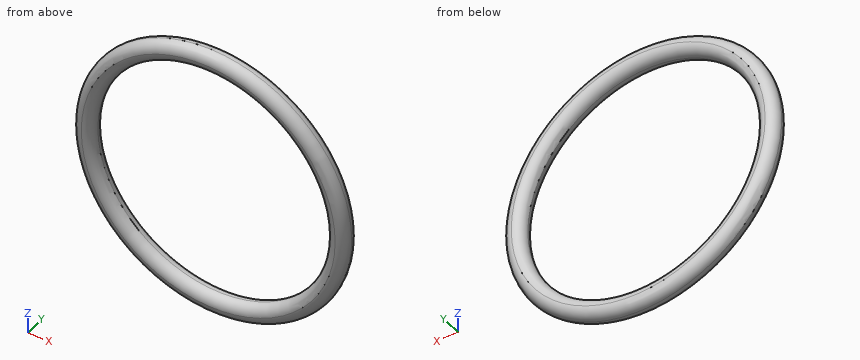
from build123d import *

# Parameters (mm, degrees)
F0_R     = 10.5
F0_R_2   = 9
F1_DEPTH = 1.5
F2_R     = 0.74999


# Not quite as in the source:
# - a fillet or chamfer is up to 0.001 mm smaller than in the source, because OpenCascade refuses the exact size


with BuildPart() as f1:
    # F0 (on Front) → F1 (new body)
    with BuildSketch(Plane.XZ):
        Circle(F0_R)
        Circle(F0_R_2, mode=Mode.SUBTRACT)
    extrude(amount=F1_DEPTH)

    # F2 (radius 0.75 in the source; OpenCascade refuses exactly that, so slightly less here)
    f2_edges = [f1.edges().sort_by_distance(p)[0] for p in [
        (-9, -1.5, 0),
        (-10.5, -1.5, 0),
        (-9, 0, 0),
        (-10.5, 0, 0),
    ]]
    fillet(f2_edges, radius=F2_R)


solid = f1.part
Could you check a few things on this model? Use its own coordinates, in mm. Give positions to 0.01 mm unless a question says otherwise; leave off trailing zeros. Loops run counter-clockwise (first coordinate to the right, second up) from the corner with the lowest first, then second, coordinate; pieces in that order, holes last. Notation, with made-up numbers: (-14.5, -37) -> (19.5, -37) arc R25 cw to (19.5, -10) -> close; hole circle Ø9 at (-26, 42). An arc over 180 degrees is marked (long way). Answer as CSV lines item,"result". Start each with the question number.
(1) I'm going to push a flat-ended pin straight in: pin 1 Ø12 at (x, z) = (-6.5, 1.5) entering from +Y. Where does the tip first touch, or does it pass through?
(2) If we section it at B-B on y = -0.5: Write out the boundary of the cut face in (x, z).
(3) I need wall thicknesses on probe 1 along Z at (x, y) = (0, -0.8); probe 2 along X at (y, z) = (-0.35, -1.75); probe 3 along Z at (x, y) = (-1, -0.1). Which ranges of each line are inside material? Lowest first, please.
Computed:
1,pin 1,"stops at y = 0"
2,outline,"circle Ø20.91 at (0, 0); hole circle Ø18.09 at (0, 0)"
3,probe 1,"z = -10.5 to -9, 9 to 10.5"
3,probe 2,"x = -10.24 to -8.95, 8.95 to 10.24"
3,probe 3,"z = -10.07 to -9.32, 9.32 to 10.07"
